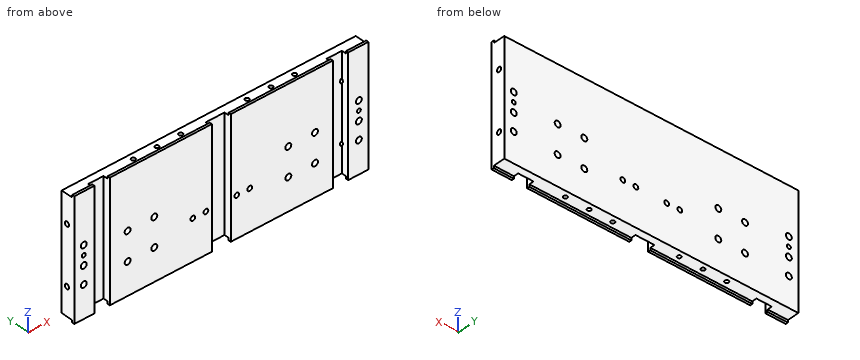
```python
from build123d import *

# Parameters (mm, degrees)
AUFSATZ_LINEAR_AUSTRAGEN1_DEPTH    = 12
SKIZZE3_W                          = 248
SKIZZE3_H                          = 2
AUFSATZ_LINEAR_AUSTRAGEN2_DEPTH    = 2
SKIZZE4_W                          = 248
SKIZZE4_H                          = 2
AUFSATZ_LINEAR_AUSTRAGEN3_DEPTH    = 2
SKIZZE5_W                          = 13
SKIZZE5_H                          = 100
SKIZZE5_W_2                        = 16
SCHNITT_LINEAR_AUSTRAGEN1_DEPTH    = 6
M4_GEWINDEBOHRUNG1_D               = 3.3
M4_GEWINDEBOHRUNG1_DEPTH           = 20
M4_GEWINDEBOHRUNG1_TIP             = 0.991420021
M4_GEWINDEBOHRUNG1_ON_FACE_2_D     = 3.3
M4_GEWINDEBOHRUNG1_ON_FACE_2_DEPTH = 20
M4_GEWINDEBOHRUNG1_ON_FACE_2_TIP   = 0.991420021
F_4_0_4_DURCHMESSER_BOHRUNG1_D     = 4
F_4_0_4_DURCHMESSER_BOHRUNG1_DEPTH = 18
F_4_0_4_DURCHMESSER_BOHRUNG1_TIP   = 1.201721238
F_4_0_4_DURCHMESSER_BOHRUNG2_D     = 4
F_4_0_4_DURCHMESSER_BOHRUNG2_DEPTH = 18
F_4_0_4_DURCHMESSER_BOHRUNG2_TIP   = 1.201721238
M4_GEWINDEBOHRUNG2_D               = 3.3
SKIZZE15_R                         = 2
SCHNITT_LINEAR_AUSTRAGEN2_DEPTH    = 135.238593556
F_5_0_5_DURCHMESSER_BOHRUNG1_D     = 5


with BuildPart() as part:
    # Skizze2 → Aufsatz-Linear austragen1 (new body)
    with BuildSketch(Plane(origin=(0, 0, 0), x_dir=(1, 0, 0), z_dir=(0, 1, 0))):
        Polygon((124, 0), (0, 0), (-124, 0), (-124, -48), (124, -48), align=None)
        Polygon((-124, 0), (0, 0), (124, 0), (124, 48), (-124, 48), align=None)
    extrude(amount=AUFSATZ_LINEAR_AUSTRAGEN1_DEPTH)

    # Skizze3 → Aufsatz-Linear austragen2 (add)
    with BuildSketch(Plane.XY.offset(48)):
        with Locations((0, 1)):
            Rectangle(SKIZZE3_W, SKIZZE3_H)
    extrude(amount=AUFSATZ_LINEAR_AUSTRAGEN2_DEPTH)

    # Skizze4 → Aufsatz-Linear austragen3 (add)
    with BuildSketch(Plane(origin=(0, 0, -48), x_dir=(-1, 0, 0), z_dir=(0, 0, -1))):
        with Locations((0, 1)):
            Rectangle(SKIZZE4_W, SKIZZE4_H)
    extrude(amount=AUFSATZ_LINEAR_AUSTRAGEN3_DEPTH)

    # Skizze5 → Schnitt-Linear austragen1 (cut)
    with BuildSketch(Plane.XZ):
        with Locations((100.5, 0)):
            Rectangle(SKIZZE5_W, SKIZZE5_H)
        Rectangle(SKIZZE5_W_2, SKIZZE5_H)
        with Locations((-100.5, 0)):
            Rectangle(SKIZZE5_W, SKIZZE5_H)
    extrude(amount=-SCHNITT_LINEAR_AUSTRAGEN1_DEPTH, mode=Mode.SUBTRACT)

    # M4 Gewindebohrung1
    with Locations(Plane(origin=(68, 7, -48), x_dir=(-1, 0, 0), z_dir=(0, 0, -1))):
        with Locations((0, 0), (20, 0), (40, 0), (136, 0), (116, 0), (96, 0)):
            Hole(M4_GEWINDEBOHRUNG1_D / 2, depth=M4_GEWINDEBOHRUNG1_DEPTH)
            with Locations((0, 0, -(M4_GEWINDEBOHRUNG1_DEPTH + M4_GEWINDEBOHRUNG1_TIP / 2))):  # 118° drill point
                Cone(0, M4_GEWINDEBOHRUNG1_D / 2, M4_GEWINDEBOHRUNG1_TIP, mode=Mode.SUBTRACT)

    # M4 Gewindebohrung1 on face 2
    with Locations(Plane(origin=(-68, 7, 48), x_dir=(1, 0, 0), z_dir=(0, 0, 1))):
        with Locations((0, 0), (20, 0), (40, 0), (136, 0), (116, 0), (96, 0)):
            Hole(M4_GEWINDEBOHRUNG1_ON_FACE_2_D / 2, depth=M4_GEWINDEBOHRUNG1_ON_FACE_2_DEPTH)
            with Locations((0, 0, -(M4_GEWINDEBOHRUNG1_ON_FACE_2_DEPTH + M4_GEWINDEBOHRUNG1_ON_FACE_2_TIP / 2))):  # 118° drill point
                Cone(0, M4_GEWINDEBOHRUNG1_ON_FACE_2_D / 2, M4_GEWINDEBOHRUNG1_ON_FACE_2_TIP, mode=Mode.SUBTRACT)

    # Ø4.0 (4) Durchmesser Bohrung1
    with Locations(Plane(origin=(-124, 7, -24.5), x_dir=(0, 0, -1), z_dir=(-1, 0, 0))):
        with Locations((0, 0), (-49, 0)):
            Hole(F_4_0_4_DURCHMESSER_BOHRUNG1_D / 2, depth=F_4_0_4_DURCHMESSER_BOHRUNG1_DEPTH)
            with Locations((0, 0, -(F_4_0_4_DURCHMESSER_BOHRUNG1_DEPTH + F_4_0_4_DURCHMESSER_BOHRUNG1_TIP / 2))):  # 118° drill point
                Cone(0, F_4_0_4_DURCHMESSER_BOHRUNG1_D / 2, F_4_0_4_DURCHMESSER_BOHRUNG1_TIP, mode=Mode.SUBTRACT)

    # Ø4.0 (4) Durchmesser Bohrung2
    with Locations(Plane(origin=(124, 7, 24.5), x_dir=(0, 0, 1), z_dir=(1, 0, 0))):
        with Locations((0, 0), (-49, 0)):
            Hole(F_4_0_4_DURCHMESSER_BOHRUNG2_D / 2, depth=F_4_0_4_DURCHMESSER_BOHRUNG2_DEPTH)
            with Locations((0, 0, -(F_4_0_4_DURCHMESSER_BOHRUNG2_DEPTH + F_4_0_4_DURCHMESSER_BOHRUNG2_TIP / 2))):  # 118° drill point
                Cone(0, F_4_0_4_DURCHMESSER_BOHRUNG2_D / 2, F_4_0_4_DURCHMESSER_BOHRUNG2_TIP, mode=Mode.SUBTRACT)

    # M4 Gewindebohrung2 (through all)
    with Locations(Plane(origin=(-116, 12, 0), x_dir=(0, 0, 1), z_dir=(0, 1, 0))):
        with Locations((0, 0), (0, 232)):
            Hole(M4_GEWINDEBOHRUNG2_D / 2)

    # Skizze15 → Schnitt-Linear austragen2 (cut, through all)
    with BuildSketch(Plane(origin=(0, 12, 0), x_dir=(1, 0, 0), z_dir=(0, 1, 0))):
        with Locations(Location((24, 16, 0), (0, 0, 270))):
            Circle(SKIZZE15_R)
        with Locations(Location((-13, 16, 0), (0, 0, 270))):
            Circle(SKIZZE15_R)
        with Locations(Location((-24, 16, 0), (0, 0, 270))):
            Circle(SKIZZE15_R)
        with Locations(Location((13, 16, 0), (0, 0, 270))):
            Circle(SKIZZE15_R)
    extrude(amount=-SCHNITT_LINEAR_AUSTRAGEN2_DEPTH, mode=Mode.SUBTRACT)

    # Ø5.0 (5) Durchmesser Bohrung1 (through all)
    with Locations(Plane(origin=(-116, 12, -23), x_dir=(0, 0, 1), z_dir=(0, 1, 0))):
        with Locations((0, 0), (31, 0), (15, 0), (24, 37), (24, 59.5), (0, 59.5), (0, 37), (0, 195), (0, 172.5), (24, 172.5), (24, 195), (31, 232), (15, 232), (0, 232)):
            Hole(F_5_0_5_DURCHMESSER_BOHRUNG1_D / 2)


solid = part.part
```
Check sheet for the modelled part. Datum: model origin and axes. Units: mm. Give positions to 0.01 mm unless a question says otherwise; leave off trailing zeros. Loops run counter-clockwise (first coordinate to the right, second up) from the corner with the lowest first, then second, coordinate; pieces in that order, holes last. Notation, with made-up numbers: M 25.25,27.5 L 78.25,27.5 A17 cw 78.25,60.5 Z; hole C 35.5,17 d9. An arc over 180 degrees is marked long. Answer in a Markdown table with one row per item.
1) Cross-section at A-A (z = 8). Enter the section's corners in (x, y).
Solutions:
| item | result |
|---|---|
| outline | M -124,0 L -118.5,0 L -118.5,12 L -124,12 Z; M -113.5,0 L -107,0 L -107,6 L -94,6 L -94,0 L -8,0 L -8,6 L 8,6 L 8,0 L 94,0 L 94,6 L 107,6 L 107,0 L 113.5,0 L 113.5,12 L -113.5,12 Z; M 118.5,0 L 124,0 L 124,12 L 118.5,12 Z |
2) Cross-section at C-C (x = 41). Enter the section's corners in (y, z).
Solutions:
| item | result |
|---|---|
| outline | M 0,-50 L 2,-50 L 2,-48 L 12,-48 L 12,48 L 2,48 L 2,50 L 0,50 Z |
3) Thickness scan on line 1 (X direction, y = 8, z = 8); line 2 (X direction, y = 1.5, z = 27); line 3 (X direction, y = 3, z = -8). Record the ranges inside material, lowest first.
Solutions:
| item | result |
|---|---|
| line 1 | x = -124 to -118.5, -113.5 to 113.5, 118.5 to 124 |
| line 2 | x = -124 to -107, -94 to -8, 8 to 94, 107 to 124 |
| line 3 | x = -124 to -118.5, -113.5 to -107, -94 to -8, 8 to 94, 107 to 113.5, 118.5 to 124 |
4) Cross-section at B-B (z = -41.5). Enter the section's corners in (x, y).
Solutions:
| item | result |
|---|---|
| outline | M -124,0 L -107,0 L -107,6 L -94,6 L -94,0 L -8,0 L -8,6 L 8,6 L 8,0 L 94,0 L 94,6 L 107,6 L 107,0 L 124,0 L 124,12 L -124,12 Z; hole C -68,7 d3.3; hole C -48,7 d3.3; hole C -28,7 d3.3; hole C 28,7 d3.3; hole C 48,7 d3.3; hole C 68,7 d3.3 |
5) Depth check by flat-ended pin: pin 1 (0.6 mm diameter, centred on x = 31, z = -48.5, fed in from +Y); pin 2 (5 mm diameter, centred on x = -29.5, y = 7, fed in from +Z); pin 3 (1 mm diameter, centred on x = -93, y = 5, fed in from -Z). Enter the tip coordinate at first touch or a pass-through.
Solutions:
| item | result |
|---|---|
| pin 1 | stops at y = 2 |
| pin 2 | stops at z = 48 |
| pin 3 | stops at z = -48 |
6) Cross-section at D-D (x = 1). Enter the section's corners in (y, z).
Solutions:
| item | result |
|---|---|
| outline | M 6,-48 L 12,-48 L 12,48 L 6,48 Z |
